Input: part model. Units: mm. Frame: model coordinates. Face numbers are marked on the shaded views. A direction names the side the tool comes from. Round coordinates to 2 decimals unless told otherwise and drop trailing zeros. Loops run counter-clockwise (first coordinate to the right, second up) from the corner with the lowest first, then second, coordinate; pieces in that order, holes last. Notation, with made-up numbers: (29.5, 65) -> (36.5, 65) arc R17 cw to (36.5, 90) -> close; hole circle Ø10 at (-28.75, 46.5). An arc over 180 degrees is marked (long way). Answer as a JSON object with one key per item and string values.
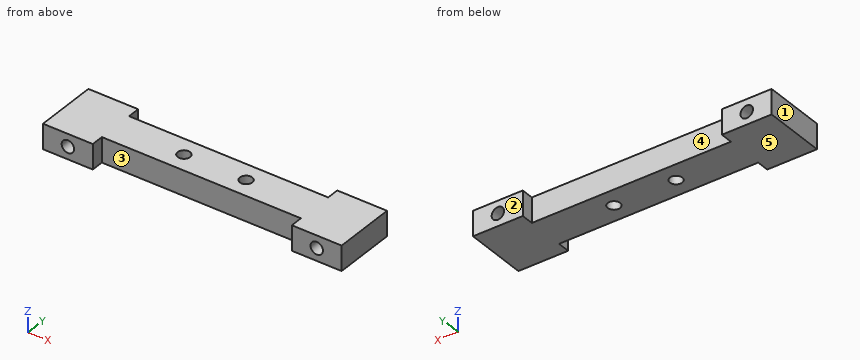
```python
from build123d import *

# Parameters (mm, degrees)
ESQUISSE1_R             = 5
BOSS_EXTRU_2_DEPTH      = 10
ESQUISSE3_R             = 5
ENL_V_MAT_EXTRU_1_DEPTH = 51


with BuildPart() as part:
    # Esquisse1 → Boss.-Extru.2 (new body, symmetric)
    with BuildSketch(Plane.XY):
        Polygon((-119.537747133, 25), (-79.537747133, 25), (-79.537747133, 15), (80.462252867, 15), (80.462252867, 25), (120.462252867, 25), (120.462252867, -25), (80.462252867, -25), (80.462252867, -15), (-79.537747133, -15), (-79.537747133, -25), (-119.537747133, -25), align=None)
        with Locations((-24.537747133, 0)):
            Circle(ESQUISSE1_R, mode=Mode.SUBTRACT)
        with Locations((25.462252867, 0)):
            Circle(ESQUISSE1_R, mode=Mode.SUBTRACT)
    extrude(amount=BOSS_EXTRU_2_DEPTH, both=True)

    # Esquisse3 → Enlèv. mat.-Extru.1 (cut, through all)
    with BuildSketch(Plane(origin=(0, 25, 0), x_dir=(1, 0, 0), z_dir=(0, 1, 0))):
        with Locations(Location((-99.537747133, 0, 0), (0, 0, 180))):  # turned: the seam where the file's is
            Circle(ESQUISSE3_R)
        with Locations(Location((100.462252867, 0, 0), (0, 0, 180))):  # turned: the seam where the file's is
            Circle(ESQUISSE3_R)
    extrude(amount=-ENL_V_MAT_EXTRU_1_DEPTH, mode=Mode.SUBTRACT)


solid = part.part
```
1) Section C-C, the plane y = 20. Output: boundary loops of the cut face in (x, z), plus the area to 3 significant figures.
Output:
{"outline": "(-119.54, -10) -> (-79.54, -10) -> (-79.54, 10) -> (-119.54, 10) -> close; (80.46, -10) -> (120.46, -10) -> (120.46, 10) -> (80.46, 10) -> close; hole circle Ø10 at (-99.54, 0); hole circle Ø10 at (100.46, 0)", "area": "1,440 mm^2"}
2) Reachability of the marked faces 4 and 5 from +Z, -Z, +X, -X, +Y, -Y: full face, straight path, thin tool, end or side. Return the list, or none.
Output:
{"face 4": "+Z, -Z, +Y", "face 5": "-Z, +X, -X, +Y, -Y"}
3) Section D-D, the plane x = -34.5. Output: boundary loops of the cut face in (y, z).
Output:
{"outline": "(-15, -10) -> (15, -10) -> (15, 10) -> (-15, 10) -> close"}
4) Ray query, probe 1 along X at (y, z) = (7, -1.75); probe 2 along X at (y, z) = (-20.5, -2); probe 3 along X at (y, z) = (18, -7.25). Return the intervals inside material, ascending.
Output:
{"probe 1": "x = -119.54 to -104.22, -94.85 to 95.78, 105.15 to 120.46", "probe 2": "x = -119.54 to -104.12, -94.96 to -79.54, 80.46 to 95.88, 105.04 to 120.46", "probe 3": "x = -119.54 to -79.54, 80.46 to 120.46"}
5) Contact query for flat-ended pins moving along their axis: P1, Ø2, axis at x = -61, y = -17, coming from the -Z side; P2, Ø1, axis at x = -69, z = 5.5, coming from the +Y side. Output: stop coordinate, or through.
Output:
{"P1": "passes through", "P2": "stops at y = 15"}
6) Section B-B, the plane z = 0. Output: boundary loops of the cut face in (x, y), plus the area to 3 significant figures.
Output:
{"outline": "(-119.54, -25) -> (-104.54, -25) -> (-104.54, 25) -> (-119.54, 25) -> close; (-94.54, -25) -> (-79.54, -25) -> (-79.54, -15) -> (80.46, -15) -> (80.46, -25) -> (95.46, -25) -> (95.46, 25) -> (80.46, 25) -> (80.46, 15) -> (-79.54, 15) -> (-79.54, 25) -> (-94.54, 25) -> close; (105.46, -25) -> (120.46, -25) -> (120.46, 25) -> (105.46, 25) -> close; hole circle Ø10 at (-24.54, 0); hole circle Ø10 at (25.46, 0)", "area": "7,640 mm^2"}
7) Section A-A, the plane y = 0. Output: boundary loops of the cut face in (x, z).
Output:
{"outline": "(-119.54, -10) -> (-29.54, -10) -> (-29.54, 10) -> (-119.54, 10) -> close; (-19.54, -10) -> (20.46, -10) -> (20.46, 10) -> (-19.54, 10) -> close; (30.46, -10) -> (120.46, -10) -> (120.46, 10) -> (30.46, 10) -> close; hole circle Ø10 at (-99.54, 0); hole circle Ø10 at (100.46, 0)"}
8) Draft query along X for the marked faces 1, 2 and 3. Return one class per face: +X half, -X half, draft (parallel to the pull), parting line (faces both ways), or undercut.
Output:
{"face 1": "-X half", "face 2": "draft", "face 3": "undercut"}
